from build123d import *

# Parameters (mm, degrees)
SKETCH5_R           = 7.9375
BOSS_EXTRUDE3_DEPTH = 50.8
CHAMFER1_SIZE       = 1.731818182
CUT_SWEEP1_PITCH    = 2.309090909
BOSS_EXTRUDE4_DEPTH = 10.715625
SKETCH8_OUTSIDE_W   = 265.784
SKETCH8_OUTSIDE_H   = 269.468
SKETCH8_OUTSIDE_R   = 11.90625
CUT_EXTRUDE3_DEPTH  = 65.147818703
CUT_EXTRUDE3_DRAFT  = -60
CUT_EXTRUDE4_DEPTH  = 0.254
CIRPATTERN1_COUNT   = 6
SKETCH13_R          = 7.9375
BOSS_EXTRUDE5_DEPTH = 51.741567


with BuildPart() as part:
    # Sketch5 → Boss-Extrude3 (new body)
    with BuildSketch(Plane(origin=(30.7578125, 0, 0), x_dir=(0, 0, -1), z_dir=(1, 0, 0))):
        Circle(SKETCH5_R)
    extrude(amount=-BOSS_EXTRUDE3_DEPTH)

    # Chamfer1
    chamfer1_edges = [part.edges().sort_by_distance(p)[0] for p in [
        (30.7578125, 0, 7.9375),
    ]]
    chamfer(chamfer1_edges, length=CHAMFER1_SIZE)

    # Cut-Sweep1: arcs per turn and ends read off the stored shape
    # Cut-Sweep1: the profile of Sketch10 profile screwed along a right-hand helix through 23 turns, 10 arcs to a turn; built about Z, then put on its axis
    cut_sweep1_z = Axis((0, 0, 0), (0, 0, 1))
    cut_sweep1_corners = [(7.9378, 0, 0.000173205), (6.43770146, 0, -0.865909091), (6.43770146, 0, -1.154545455), (7.9378, 0, -2.020627751)]
    with BuildLine(mode=Mode.PRIVATE) as cut_sweep1_profile:
        Line(cut_sweep1_corners[0], cut_sweep1_corners[1])
        Line(cut_sweep1_corners[1], cut_sweep1_corners[2])
        Line(cut_sweep1_corners[2], cut_sweep1_corners[3])
        Line(cut_sweep1_corners[3], cut_sweep1_corners[0])
    cut_sweep1_cap = Face(cut_sweep1_profile.wire())
    cut_sweep1_turn_angles = [0, 18, 36, 54, 72, 90, 108, 126, 144, 162, 180, 198, 216, 234, 252, 270, 288, 306, 324, 342, 360]
    cut_sweep1_turn_weights = [1, 0.9510565162951535, 1, 0.9510565162951535, 1, 0.9510565162951535, 1, 0.9510565162951535, 1, 0.9510565162951535, 1, 0.9510565162951535, 1, 0.9510565162951535, 1, 0.9510565162951535, 1, 0.9510565162951535, 1, 0.9510565162951535, 1]
    cut_sweep1_turn_rails = [Edge.make_bspline([Vector(p[0], p[1], 0).rotate(cut_sweep1_z, cut_sweep1_turn_angles[k]) / cut_sweep1_turn_weights[k] + Vector(0, 0, p[2] + CUT_SWEEP1_PITCH * cut_sweep1_turn_angles[k] / 360) for k in range(21)], [0, 0, 0, 1, 1, 2, 2, 3, 3, 4, 4, 5, 5, 6, 6, 7, 7, 8, 8, 9, 9, 10, 10, 10], 2, cut_sweep1_turn_weights) for p in cut_sweep1_corners]
    cut_sweep1_turn_sides = [Face.make_surface_from_curves(cut_sweep1_turn_rails[p[0]], cut_sweep1_turn_rails[p[1]]) for p in [(0, 1), (1, 2), (2, 3), (3, 0)]]
    cut_sweep1 = Plane(origin=(30.7578125, 0, 0), x_dir=(0, 1, 0), z_dir=(-1, 0, 0)) * Solid(Shell([*[p.moved(Location((0, 0, CUT_SWEEP1_PITCH * i))) for i in range(23) for p in cut_sweep1_turn_sides], cut_sweep1_cap, cut_sweep1_cap.rotate(cut_sweep1_z, 8280).moved(Location((0, 0, CUT_SWEEP1_PITCH * 8280 / 360)))]))
    add(cut_sweep1, mode=Mode.SUBTRACT)

    # Sketch6 → Boss-Extrude4 (add)
    with BuildSketch(Plane.ZY.offset(20.0421875)):
        Polygon((11.90625, 6.874076643), (0, 13.748153285), (-11.90625, 6.874076643), (-11.90625, -6.874076643), (0, -13.748153285), (11.90625, -6.874076643), align=None)
    extrude(amount=BOSS_EXTRUDE4_DEPTH)


with BuildPart() as cut_extrude3_tool:
    # Sketch8 outside → Cut-Extrude3 (with draft: the straight prism first)
    with BuildSketch(Plane.ZY.offset(30.7578125)):
        Rectangle(SKETCH8_OUTSIDE_W, SKETCH8_OUTSIDE_H)
        Circle(SKETCH8_OUTSIDE_R, mode=Mode.SUBTRACT)
    extrude(amount=-CUT_EXTRUDE3_DEPTH)
    # Cut-Extrude3: the draft: its side faces are tilted about the plane it starts from
    cut_extrude3_sides = [cut_extrude3_tool.faces().sort_by_distance(p)[0] for p in [
        (1.816096852, -134.734, 0),
        (1.816096852, 0, 132.892),
        (1.816096852, 134.734, 0),
        (1.816096852, 0, -132.892),
        (1.816096852, 0, -11.90625),
    ]]
    draft(cut_extrude3_sides, Plane.ZY.offset(30.7578125), CUT_EXTRUDE3_DRAFT)


with BuildPart() as part_1:
    add(part.part)

    # Cut-Extrude3: cut by cut_extrude3_tool
    add(cut_extrude3_tool.part, mode=Mode.SUBTRACT)

    # Sketch12 → Cut-Extrude4 (cut)
    with BuildSketch(Plane.ZY.offset(30.7578125)):
        with BuildLine():
            Line((0.3571875, 9.1678125), (0.3571875, 5.1196875))
            ThreePointArc((0.3571875, 5.1196875), (0, 4.7625), (-0.3571875, 5.1196875))
            Line((-0.3571875, 5.1196875), (-0.3571875, 9.1678125))
            ThreePointArc((-0.3571875, 9.1678125), (0, 9.525), (0.3571875, 9.1678125))
        make_face()
    cut_extrude4 = extrude(amount=-CUT_EXTRUDE4_DEPTH, mode=Mode.SUBTRACT)

    # CirPattern1: Cut-Extrude4 ×6 about axis
    cirpattern1_axis = Axis((0, 0, 0), (1, 0, 0))
    for i in range(1, CIRPATTERN1_COUNT):
        add(cut_extrude4.rotate(cirpattern1_axis, i * 360 / CIRPATTERN1_COUNT), mode=Mode.SUBTRACT)

    # Sketch13 → Boss-Extrude5 (add)
    with BuildSketch(Plane(origin=(-20.0421875, 0, 0), x_dir=(0, 0, -1), z_dir=(1, 0, 0))):
        Circle(SKETCH13_R)
    extrude(amount=BOSS_EXTRUDE5_DEPTH)


solid = part_1.part
Work out the finished part from the listing and answer in its coordinate system (mm). A direction names the side the tool comes from. Coordinates: 2 decimals unless noted, no trailing zeros. Loops run counter-clockwise (first coordinate to the right, second up) from the corner with the lowest first, then second, coordinate; pieces in that order, holes last. Notation, with made-up numbers: (-19.5, 79.25) -> (-5.5, 79.25) arc R16 ccw to (-5.5, 110.25) -> close; hole circle Ø3 at (39, -1.5). An arc over 180 degrees is marked (long way). Write each question's results on one line, items separated by ' | '. Start each with the question number.
1) The mould has two halves that part along Z. Classify faces 1 (the flat face through (-30.504, -3.6, -6.2)), 2 (the conical face through (-30.5, 6.15, 10.71)), 3 (the flat face through (31.699, 0, 0)): pulls with the +Z half, pulls with the -Z half, needs draft (parallel to the pull), parting line crosses it, or undercut.
2) Consider line 1 along X through (y, z) = (-10.25, 1.25); line 2 along Y through (x, z) = (-13, 5.25); line 3 along Z through (x, y) = (11.5, -7). Determine where each line is inside the solid, lowest interval first.
3) Find section A-A on x = -21. Determine the outline of the cut face in (y, z), then the cut area to 3 significant figures.
4) For faces 4 (the flat face through (-30.504, -3.6, 6.2)), 5 (the flat face through (-25.32, -10.36, 5.87)), determine the directions among +Z, -Z, +X, -X, +Y, -Y from which every point of the face is accessible in a straight line to the end or side of a thin tool.
5) Find section B-B on x = 23. Determine the outline of the cut face in (y, z) (1 decimal).
6) Flat-ended cylindrical pins translate along their axes: P1, Ø3, axis at x = -10, z = 5.5, coming from the -Y side; P2, Ø3, axis at x = 23, y = -9.5, coming from the +Z side; P3, Ø6, axis at x = 2, y = 5, coming from the -Z side; P4, Ø8, axis at x = 17.5, y = -0.5, coming from the -Z side. Find the tip coordinate at first contact, or state that the pin passes through.
Response values:
1) face 1: undercut | face 2: pulls with the +Z half | face 3: needs draft
2) line 1: x = -30.76 to -20.04 | line 2: y = -5.95 to 5.95 | line 3: z = -3.74 to 3.74
3) outline: (-13.75, 0) -> (-6.87, -11.91) -> (6.87, -11.91) -> (13.75, 0) -> (6.87, 11.91) -> (-6.87, 11.91) -> close | area: 491 mm^2
4) face 4: -X | face 5: +Z, +X, -X, -Y
5) outline: circle Ø15.9 at (0, 0)
6) P1: stops at y = -6.86 | P2: passes through | P3: stops at z = -7.68 | P4: stops at z = -7.94
